Here's how the part is built. I have some questions about the finished solid (model axes, mm). Face numbers are marked on the shaded views. A direction names the side the tool comes from. Round coordinates to 2 decimals unless told otherwise and drop trailing zeros. Order: outer loops, then holes, each group sorted by start corner. A loop starts at its lowest first (then second) coordinate and runs counter-clockwise, first axis right, second up.
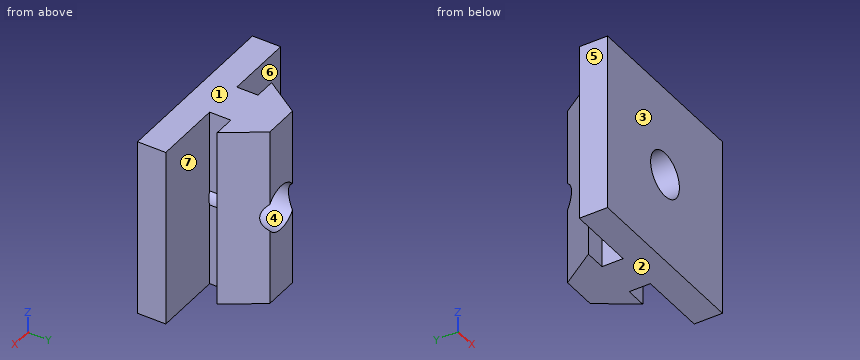
```python
from build123d import *

# Parameters (mm, degrees)
BOSS_EXTRUDE1_DEPTH = 25.34
SKETCH2_R           = 3.175
CUT_EXTRUDE1_DEPTH  = 31.848196463


with BuildPart() as part:
    # Sketch1 → Boss-Extrude1 (new body)
    with BuildSketch(Plane.XY):
        Polygon((12.675, 0), (-12.675, 0), (-12.675, 4), (-3, 4), (-3, 7), (-6, 7), (-2.5, 12.2), (2.5, 12.2), (6, 7), (3, 7), (3, 4), (12.675, 4), align=None)
    extrude(amount=BOSS_EXTRUDE1_DEPTH)

    # Sketch2 → Cut-Extrude1 (cut, through all)
    with BuildSketch(Plane.XZ):
        with Locations(Location((0, 12.67, 0), (0, 0, 270))):
            Circle(SKETCH2_R)
    extrude(amount=-CUT_EXTRUDE1_DEPTH, mode=Mode.SUBTRACT)


solid = part.part
```
1. If we section it at A-A, the plane x = 0: Write out the boundary of the cut face in (y, z) (3 decimals), and give its area (3 significant figures).
Evaluation:
outline: (0, 0) - (12.2, 0) - (12.2, 9.495) - (0, 9.495) - close; (0, 15.845) - (12.2, 15.845) - (12.2, 25.34) - (0, 25.34) - close
area: 232 mm2
2. If we section it at D-D, the plane y = 1: Write out the boundary of the cut face in (x, z) (3 decimals), and give its area (3 significant figures).
Evaluation:
outline: (-12.675, 0) - (12.675, 0) - (12.675, 25.34) - (-12.675, 25.34) - close; hole circle Ø6.35 at (0, 12.67)
area: 611 mm2
3. On a 3-axis mill with a long thin cutter (end or side, diameter ignored), from which of +Z, -Z, +X, -X, +Y, -Y can I reach the whole of each face in a straight line? I mean the marked faces 5, 6 and 7. Say none if no direction works.
Evaluation:
face 5: +Z, -Z, -X, +Y, -Y
face 6: +Z, -Z, -X
face 7: +Z, -Z, +X
4. I'm going to push flat-ended pins straight in: P1, Ø1.5, axis at y = 5.5, z = 18.5, coming from the +X side; P2, Ø5, axis at x = 0, z = 12.67, coming from the -Y side; P3, Ø1.5, axis at y = 10, z = 7, coming from the -X side; P4, Ø3.5, axis at y = 6, z = 5.5, coming from the +X side. Where does each tip first touch, or does it pass through?
Evaluation:
P1: stops at x = 3
P2: passes through
P3: stops at x = -4.49
P4: stops at x = 6
5. I need wall thicknesses on probe 1 along Z at (x, y) = (0, 7) (3 decimals); probe 2 along X at (y, z) = (3.25, 12.67) (3 decimals); probe 3 along X at (y, z) = (5.75, 22.5). Which ranges of each line are inside material? Lowest first, please.
Evaluation:
probe 1: z = 0 to 9.495, 15.845 to 25.34
probe 2: x = -12.675 to -3.175, 3.175 to 12.675
probe 3: x = -3 to 3
6. If we section it at C-C, the plane z = 12.67: Write out the boundary of the cut face in (x, y) (3 decimals).
Evaluation:
outline: (-12.675, 0) - (-3.175, 0) - (-3.175, 4) - (-12.675, 4) - close; (-6, 7) - (-3.175, 7) - (-3.175, 11.197) - close; (3.175, 0) - (12.675, 0) - (12.675, 4) - (3.175, 4) - close; (3.175, 7) - (6, 7) - (3.175, 11.197) - close
7. If we section it at B-B, the plane y = 6.25: Write out the boundary of the cut face in (x, z) (3 decimals).
Evaluation:
outline: (-3, 0) - (3, 0) - (3, 11.63) arc R3.175 cw to (-3, 11.63) - close; (-3, 13.71) arc R3.175 cw to (3, 13.71) - (3, 25.34) - (-3, 25.34) - close
8. If we mould it in two halves opening along Z, with no side actions, what happens to the marked faces 1, 2, 3 and 4? For each: released by +Z, released by -Z, zero draft, split by the parting line, or undercut.
Evaluation:
face 1: released by +Z
face 2: released by -Z
face 3: zero draft
face 4: undercut
